Could you check a few things on this model? Use its own coordinates, in mm. A direction names the side the tool comes from. Round coordinates to 2 decimals unless told otherwise and drop trailing zeros. Loops run counter-clockwise (first coordinate to the right, second up) from the corner with the lowest first, then second, coordinate; pieces in that order, holes last. Notation, with made-up numbers: M -2.5,17.25 L 2.5,17.25 A9 ccw 2.5,33.25 Z; hole C 60.25,-14 d10. An arc over 180 degrees is marked long. Answer in a Markdown table with one row per item.
Autodesk Inventor part; units mm, degrees
ref_plane "YZ Plane" through (0, 0, 0) normal (1, 0, 0) x (0, 1, 0)
ref_plane "XZ Plane" through (0, 0, 0) normal (0, 1, 0) x (-1, 0, 0)
ref_plane "XY Plane" through (0, 0, 0) normal (0, 0, 1) x (1, 0, 0)
sketch "Sketch1" plane through (0, 0, 0) normal (0, 0, 1) x (1, 0, 0)
  circle A0 centre (0, 0) radius 31.75
  line L0 (-24.9602, 8.8198) -> (23.1368, 8.8198) construction
  line L1 (23.1368, 8.8198) -> (23.1368, -14.9885) construction
  line L2 (23.1368, -14.9885) -> (-24.9602, -14.9885) construction
  line L3 (-24.9602, -14.9885) -> (-24.9602, 8.8198) construction
  line L4 (-13.7341, 8.4322) -> (-13.7341, 5.3888)
  line L5 (-13.7341, 5.3888) -> (-19.6343, 5.3888)
  line L6 (-19.6343, 5.3888) -> (-19.6343, 2.1444)
  spline S0 degree 2 poles (-19.6343, 2.1444) (-18.5289, 3.4507) (-16.7775, 3.4507) knots 0 0 0 1 1 1
  spline S1 degree 2 poles (-16.7775, 3.4507) (-14.8107, 3.4507) (-12.8009, 1.2543) (-12.8009, -1.8752) knots 0 0 0 1 2 2 2
  line L7 (-12.8009, -1.8752) -> (-12.8009, -4.5884)
  spline S2 degree 2 poles (-12.8009, -4.5884) (-12.8009, -6.6126) (-13.1886, -8.5076) (-14.4662, -10.1154) (-16.7344, -10.9767) (-18.371, -10.9767) knots 0 0 0 1 2 3 4 4 4
  spline S3 degree 2 poles (-18.371, -10.9767) (-20.2085, -10.9767) (-23.0078, -9.6991) (-24.185, -7.1581) (-24.185, -4.5023) knots 0 0 0 1 2 3 3 3
  line L8 (-24.185, -4.5023) -> (-24.185, -3.4687)
  line L9 (-24.185, -3.4687) -> (-19.4333, -3.4687)
  line L10 (-19.4333, -3.4687) -> (-19.4333, -4.6602)
  spline S4 degree 2 poles (-19.4333, -4.6602) (-19.4333, -6.4978) (-19.1749, -8.0482) (-18.3997, -8.0482) knots 0 0 0 1 2 2 2
  spline S5 degree 2 poles (-18.3997, -8.0482) (-18.0551, -8.0482) (-17.6101, -7.6031) (-17.5814, -7.0863) (-17.5527, -5.0909) knots 0 0 0 1 2 3 3 3
  line L11 (-17.5527, -5.0909) -> (-17.5527, -1.3297)
  spline S6 degree 2 poles (-17.5527, -1.3297) (-17.5527, -0.253) (-17.9977, 0.5222) (-18.5289, 0.5222) knots 0 0 0 1 2 2 2
  spline S7 degree 2 poles (-18.5289, 0.5222) (-18.859, 0.5222) (-19.3041, 0.1202) (-19.4333, -0.3392) (-19.4333, -1.1718) knots 0 0 0 1 2 3 3 3
  line L12 (-19.4333, -1.1718) -> (-24.1419, -1.1718)
  line L13 (-24.1419, -1.1718) -> (-23.941, 8.4322)
  line L14 (-23.941, 8.4322) -> (-13.7341, 8.4322)
  line L15 (0.234, 3.379) -> (-4.5177, 3.379)
  spline S8 degree 2 poles (-4.5177, 3.379) (-4.5177, 4.714) (-4.5751, 5.4031) (-5.0776, 5.8768) (-5.5226, 5.8768) knots 0 0 0 1 2 3 3 3
  spline S9 degree 2 poles (-5.5226, 5.8768) (-5.8815, 5.8768) (-6.3552, 5.4318) (-6.427, 4.7284) (-6.427, 3.6517) knots 0 0 0 1 2 3 3 3
  line L16 (-6.427, 3.6517) -> (-6.427, 0.6083)
  spline S10 degree 2 poles (-6.427, 0.6083) (-6.0681, 1.3835) (-4.6469, 2.1444) (-3.6133, 2.1444) knots 0 0 0 1 2 2 2
  spline S11 degree 2 poles (-3.6133, 2.1444) (-2.3069, 2.1444) (-0.3115, 0.7375) (0.234, -1.2436) (0.234, -2.9232) knots 0 0 0 1 2 3 3 3
  line L17 (0.234, -2.9232) -> (0.234, -4.4449)
  spline S12 degree 2 poles (0.234, -4.4449) (0.234, -6.4403) (-0.0675, -8.3927) (-1.4025, -10.058) (-3.7138, -10.9767) (-5.2642, -10.9767) knots 0 0 0 1 2 3 4 4 4
  spline S13 degree 2 poles (-5.2642, -10.9767) (-7.1735, -10.9767) (-9.6283, -9.9144) (-10.9491, -7.9333) (-11.1788, -5.7369) (-11.1788, -2.5787) knots 0 0 0 1 2 3 4 4 4
  line L18 (-11.1788, -2.5787) -> (-11.1788, 0.0484)
  spline S14 degree 2 poles (-11.1788, 0.0484) (-11.1788, 3.4507) (-10.9778, 5.7476) (-9.5422, 7.8005) (-7.0587, 8.8198) (-5.4365, 8.8198) knots 0 0 0 1 2 3 4 4 4
  spline S15 degree 2 poles (-5.4365, 8.8198) (-3.441, 8.8198) (-0.8714, 7.5278) (0.234, 5.1734) (0.234, 3.379) knots 0 0 0 1 2 3 3 3
  spline S16 degree 2 poles (-4.5177, -2.5643) (-4.5177, -1.545) (-4.9627, -0.7985) (-5.4652, -0.7985) knots 0 0 0 1 2 2 2
  spline S17 degree 2 poles (-5.4652, -0.7985) (-5.9676, -0.7985) (-6.427, -1.5163) (-6.427, -2.5643) knots 0 0 0 1 2 2 2
  line L19 (-6.427, -2.5643) -> (-6.427, -6.0097)
  spline S18 degree 2 poles (-6.427, -6.0097) (-6.427, -7.273) (-5.9964, -8.0482) (-5.4795, -8.0482) knots 0 0 0 1 2 2 2
  spline S19 degree 2 poles (-5.4795, -8.0482) (-5.1781, -8.0482) (-4.5177, -7.4452) (-4.5177, -6.1245) knots 0 0 0 1 2 2 2
  line L20 (-4.5177, -6.1245) -> (-4.5177, -2.5643)
  line L21 (9.192, 8.4322) -> (9.192, -10.6178)
  line L22 (9.192, -10.6178) -> (4.4402, -10.6178)
  line L23 (4.4402, -10.6178) -> (4.4402, -0.3966)
  spline S20 degree 2 poles (4.4402, -0.3966) (4.4402, 1.8142) (4.2249, 2.7042) (3.2774, 3.1636) (1.6409, 3.1636) knots 0 0 0 1 2 3 3 3
  line L24 (1.6409, 3.1636) -> (1.1671, 3.1636)
  line L25 (1.1671, 3.1636) -> (1.1671, 5.3888)
  spline S21 degree 2 poles (1.1671, 5.3888) (4.6125, 6.1209) (6.407, 8.4322) knots 0 0 0 1 1 1
  line L26 (6.407, 8.4322) -> (9.192, 8.4322)
  spline S22 degree 2 poles (20.1166, 0.2064) (21.1646, -0.2243) (22.2987, -1.9039) (22.2987, -5.0765) knots 0 0 0 1 2 2 2
  spline S23 degree 2 poles (22.2987, -5.0765) (22.2987, -7.3878) (21.4087, -9.5699) (18.8103, -10.9767) (16.6426, -10.9767) knots 0 0 0 1 2 3 3 3
  spline S24 degree 2 poles (16.6426, -10.9767) (14.5179, -10.9767) (12.0487, -9.6273) (10.9721, -7.4165) (10.9721, -4.8469) knots 0 0 0 1 2 3 3 3
  spline S25 degree 2 poles (10.9721, -4.8469) (10.9721, -3.1098) (11.5032, -0.5689) (12.9101, 0.2064) knots 0 0 0 1 2 2 2
  spline S26 degree 2 poles (12.9101, 0.2064) (12.02, 0.6227) (11.1443, 2.4746) (11.1443, 3.8958) knots 0 0 0 1 2 2 2
  spline S27 degree 2 poles (11.1443, 3.8958) (11.1443, 6.3506) (13.8719, 8.8054) (16.5851, 8.8054) knots 0 0 0 1 2 2 2
  spline S28 degree 2 poles (16.5851, 8.8054) (19.729, 8.8054) (22.1264, 6.1927) (22.1264, 3.7666) knots 0 0 0 1 2 2 2
  spline S29 degree 2 poles (22.1264, 3.7666) (22.1264, 2.2305) (21.3369, 0.8667) (20.1166, 0.2064) knots 0 0 0 1 2 2 2
  spline S30 degree 2 poles (17.547, -3.6266) (17.547, -2.5356) (17.102, -1.8178) (16.6139, -1.8178) knots 0 0 0 1 2 2 2
  spline S31 degree 2 poles (16.6139, -1.8178) (16.1401, -1.8178) (15.7238, -2.5069) (15.7238, -3.6266) knots 0 0 0 1 2 2 2
  line L27 (15.7238, -3.6266) -> (15.7238, -6.1102)
  spline S32 degree 2 poles (15.7238, -6.1102) (15.7238, -7.3447) (16.1832, -8.0482) (16.6856, -8.0482) knots 0 0 0 1 2 2 2
  spline S33 degree 2 poles (16.6856, -8.0482) (17.1881, -8.0482) (17.547, -7.3304) (17.547, -6.0671) knots 0 0 0 1 2 2 2
  line L28 (17.547, -6.0671) -> (17.547, -3.6266)
  spline S34 degree 2 poles (17.4465, 4.2834) (17.4465, 5.2596) (17.102, 5.8768) (16.6282, 5.8768) knots 0 0 0 1 2 2 2
  spline S35 degree 2 poles (16.6282, 5.8768) (16.1545, 5.8768) (15.8243, 5.2021) (15.8243, 4.2834) knots 0 0 0 1 2 2 2
  line L29 (15.8243, 4.2834) -> (15.8243, 2.8478)
  spline S36 degree 2 poles (15.8243, 2.8478) (15.8243, 1.9865) (16.1975, 1.3261) (16.6426, 1.3261) knots 0 0 0 1 2 2 2
  spline S37 degree 2 poles (16.6426, 1.3261) (17.1163, 1.3261) (17.4465, 1.9721) (17.4465, 2.9914) knots 0 0 0 1 2 2 2
  line L30 (17.4465, 2.9914) -> (17.4465, 4.2834)
  dimension "d0" = 63.5
extrude "Extrusion1" add sketch "Sketch1" along normal blind 1.2 contours A0 | L4 L5 L6 S0 S1 L7 S2 S3 L8 L9 L10 S4 S5 L11 S6 S7 L12 L13 L14 | L15 S8 S9 L16 S10 S11 L17 S12 S13 L18 S14 S15 | L20 S19 S18 L19 S17 S16 | L21 L22 L23 S20 L24 L25 S21 L26 | S22 S23 S24 S25 S26 S27 S28 S29 | L28 S33 S32 L27 S31 S30 | L30 S37 S36 L29 S35 S34
extrude "Extrusion2" cut sketch "Sketch1" against normal blind 0.6 from surface at 1.2 contours L4 L5 L6 S0 S1 L7 S2 S3 L8 L9 L10 S4 S5 L11 S6 S7 L12 L13 L14 | L15 S8 S9 L16 S10 S11 L17 S12 S13 L18 S14 S15 | L21 L22 L23 S20 L24 L25 S21 L26 | S22 S23 S24 S25 S26 S27 S28 S29
properties part number "Blue Alliance Marker 5618"
1) Will these pins go through, and if not, where does the flat tip stop? P1, Ø0.5, axis at x = -17.5, z = 1, coming from the -Y side; P2, Ø0.5, axis at y = -3.5, z = 1, coming from the -X side; P3, Ø0.7, axis at y = -4, z = 1, coming from the +X side.
Computed:
| item | result |
|---|---|
| P1 | stops at y = -26.66 |
| P2 | stops at x = -31.58 |
| P3 | stops at x = 31.54 |
2) Which directions (+Z, -Z, +X, -X, +Y, -Y) give clear straight access to the entire face, cutting with the end or side of a thin tool? Please do faces 1 (the face through (-20, -1, 0.6)), 2 (the face through (17, 4, 1.2)).
Computed:
| item | result |
|---|---|
| face 1 | +Z |
| face 2 | +Z, +X, -X, +Y, -Y |
3) I need wall thicknesses on line 1 (X direction, y = 6, z = 1); line 2 (Y direction, x = -22, z = 0.85); line 3 (Y direction, x = -23, z = 0.8). Which ranges of each line are inside material? Lowest first, please.
Computed:
| item | result |
|---|---|
| line 1 | x = -31.18 to -23.99, -13.73 to -10.71, -0.17 to 3.16, 9.19 to 11.47, 21.8 to 31.18 |
| line 2 | y = -22.89 to -10.14, -3.47 to -1.17, 8.43 to 22.89 |
| line 3 | y = -21.89 to -9.34, -3.47 to -1.17, 8.43 to 21.89 |
4) I want a section at B-B, the plane y = -19. Please give me the cut outline in (x, z), plus the area to 3 significant figures.
Computed:
| item | result |
|---|---|
| outline | M -25.44,0 L 25.44,0 L 25.44,1.2 L -25.44,1.2 Z |
| area | 61.0 mm² |
5) I want a section at A-A, the plane z = 0.85. State how many separate pieces and enclosed holes the cut face has, plus the area to 3 significant figures.
Computed:
| item | result |
|---|---|
| separate pieces | 4 |
| enclosed holes | 4 |
| area | 2,550 mm² |
6) If we mould it in two halves opening along X, with no side actions, what happens to faces 3 (the face through (-5, -4, 1.2)), 4 (the face through (-6.883, 30.995, 0.592)), 5 (the face through (6, -1, 0.6)), 6 (the face through (17, -1, 0.6))? For each: released by +X, released by -X, zero draft, split by the parting line, or undercut.
Computed:
| item | result |
|---|---|
| face 3 | zero draft |
| face 4 | split by the parting line |
| face 5 | undercut |
| face 6 | undercut |
